The model under review builds one solid part; all positions refer to its coordinate system, in mm. A direction names the side the tool comes from. Round coordinates to 2 decimals unless told otherwise and drop trailing zeros. Write each loop counter-clockwise with the first axis right and the second up, starting at its lowest first coordinate (ties: lowest second). Pieces come first, ordered by that corner, then holes.
Item 1: Machinability: for faces 4 (the face through (3.233, -1.341, 31.627)), 5 (the face through (-1.5, 0, 33)), which of the approach directions +Z, -Z, +X, -X, +Y, -Y give a long, thin tool a straight path to every point of the face, cutting with its end or side? Answer none if there is none.
Item 2: Add section B-B (z = 16.5). Give the boundary of the cut face in (x, y).
Item 3: To check wall thickness, follow L1, parallel to Y at x = 0, z = 25.5; L2, parallel to Z at x = -0.25, y = 1.5; L3, parallel to Z at x = -1.25, y = -1.75. State the ranges of each line that lie inside material, in increasing order.
Item 4: Clearance check with flat-ended pins moving along their axes: pin 1 Ø2 at (y, z) = (-2.5, 8.5) entering from -X; pin 2 Ø1.5 at (y, z) = (1.5, 15.5) entering from +X; pin 3 Ø1 at (y, z) = (2, 13) entering from +X. State where each tip first meets the part, or that it passes through.
Item 5: Draft analysis for pull direction Y (two halves, no side actions). For faces 1 (the face through (2, -2, 30)), 2 (the face through (-0.76, -1.293, 32.768)), 3 (the face through (0, -2, 15)), state which applies: +Y half, -Y half, draft (parallel to the pull), parting line (faces both ways), or undercut.
Item 6: Add section A-A (y = 0). Give the boundary of the cut face in (x, z).
```python
from build123d import *

# Parameters (mm, degrees)
ESQUISSE1_R             = 2
BASE_EXTRUSION_DEPTH    = 30
ESQUISSE2_R             = 3.5
BOSS_EXTRU_1_DEPTH      = 4
CHANFREIN1_SIZE         = 0.4
CONG_1_R                = 0.7
ENL_V_MAT_EXTRU_1_DEPTH = 2.5


with BuildPart() as part:
    # Esquisse1 → Base-Extrusion (new body)
    with BuildSketch(Plane.XY):
        Circle(ESQUISSE1_R)
    extrude(amount=BASE_EXTRUSION_DEPTH)

    # Esquisse2 → Boss.-Extru.1 (add)
    with BuildSketch(Plane.XY.offset(30)):
        Circle(ESQUISSE2_R)
    extrude(amount=BOSS_EXTRU_1_DEPTH)

    # Chanfrein1
    chanfrein1_edges = [part.edges().sort_by_distance(p)[0] for p in [
        (-2, 0, 0),
    ]]
    chamfer(chanfrein1_edges, length=CHANFREIN1_SIZE)

    # Congé1
    cong_1_edges = [part.edges().sort_by_distance(p)[0] for p in [
        (-3.5, 0, 34),
    ]]
    fillet(cong_1_edges, radius=CONG_1_R)

    # Esquisse3 → Enlèv. mat.-Extru.1 (cut)
    with BuildSketch(Plane.XY.offset(34)):
        Polygon((0, 1.732050808), (-1.5, 0.866025404), (-1.5, -0.866025404), (0, -1.732050808), (1.5, -0.866025404), (1.5, 0.866025404), align=None)
    extrude(amount=-ENL_V_MAT_EXTRU_1_DEPTH, mode=Mode.SUBTRACT)


solid = part.part
```
Numbers:
1. face 4: +Z, -Z
1. face 5: +Z
2. outline: circle Ø4 at (0, 0)
3. L1: y = -2 to 2
3. L2: z = 0 to 31.5
3. L3: z = 30 to 34
4. pin 1: stops at x = -1.32
4. pin 2: stops at x = 1.85
4. pin 3: stops at x = 1.32
5. face 1: draft
5. face 2: undercut
5. face 3: parting line
6. outline: (-3.5, 30) - (-2, 30) - (-2, 0.4) - (-1.6, 0) - (1.6, 0) - (2, 0.4) - (2, 30) - (3.5, 30) - (3.5, 33.3) arc R0.7 ccw to (2.8, 34) - (1.5, 34) - (1.5, 31.5) - (-1.5, 31.5) - (-1.5, 34) - (-2.8, 34) arc R0.7 ccw to (-3.5, 33.3) - close
